from build123d import *

# Parameters (mm, degrees)
SKETCH1_R           = 1.6
BOSS_EXTRUDE1_DEPTH = 6
SKETCH2_W           = 138.2
SKETCH2_H           = 67.6
SKETCH2_R           = 2.5
BOSS_EXTRUDE2_DEPTH = 3.2
FILLET1_R           = 6
FILLET2_R           = 5
FILLET3_R           = 5


with BuildPart() as part:
    # Sketch1 → Boss-Extrude1 (new body)
    with BuildSketch(Plane.XY):
        with BuildLine():
            Line((0, 21.6), (-6, 21.6))
            ThreePointArc((-6, 21.6), (-9.6, 18), (-6, 14.4))
            Line((-6, 14.4), (0, 14.4))
            Line((0, 14.4), (0, 0))
            Line((0, 0), (102.2, 0))
            Line((102.2, 0), (102.2, 46))
            Line((102.2, 46), (108.2, 46))
            ThreePointArc((108.2, 46), (111.8, 49.6), (108.2, 53.2))
            Line((108.2, 53.2), (102.2, 53.2))
            Line((102.2, 53.2), (102.2, 67.6))
            Line((102.2, 67.6), (0, 67.6))
            Line((0, 67.6), (0, 21.6))
        make_face()
        with Locations((-6, 18)):
            Circle(SKETCH1_R, mode=Mode.SUBTRACT)
        with BuildLine():
            Line((94.706674091, 2.5), (7.493325909, 2.5))
            ThreePointArc((7.493325909, 2.5), (7.045584412, 7.045584412), (2.5, 7.493325909))
            Line((2.5, 7.493325909), (2.5, 65.1))
            Line((2.5, 65.1), (99.7, 65.1))
            Line((99.7, 65.1), (99.7, 57.093325909))
            ThreePointArc((99.7, 57.093325909), (94.1, 54.1), (99.7, 51.106674091))
            Line((99.7, 51.106674091), (99.7, 7.493325909))
            ThreePointArc((99.7, 7.493325909), (95.154415588, 7.045584412), (94.706674091, 2.5))
        make_face(mode=Mode.SUBTRACT)
        with Locations((108.2, 49.6)):
            Circle(SKETCH1_R, mode=Mode.SUBTRACT)
        with Locations((4.5, 4.5)):
            Circle(SKETCH1_R, mode=Mode.SUBTRACT)
        with Locations((97.7, 4.5)):
            Circle(SKETCH1_R, mode=Mode.SUBTRACT)
        with Locations((97.7, 54.1)):
            Circle(SKETCH1_R, mode=Mode.SUBTRACT)
    extrude(amount=BOSS_EXTRUDE1_DEPTH)

    # Sketch2 → Boss-Extrude2 (add)
    with BuildSketch(Plane(origin=(0, 0, 0), x_dir=(-1, 0, 0), z_dir=(0, 0, -1))):
        with Locations((-51.1, 33.8)):
            Rectangle(SKETCH2_W, SKETCH2_H)
        with Locations((-112.2, 59.6)):
            Circle(SKETCH2_R, mode=Mode.SUBTRACT)
        with Locations((-112.2, 8)):
            Circle(SKETCH2_R, mode=Mode.SUBTRACT)
        with Locations(Location((10, 8, 0), (0, 0, 180))):
            Circle(SKETCH2_R, mode=Mode.SUBTRACT)
        with Locations(Location((10, 59.6, 0), (0, 0, 180))):
            Circle(SKETCH2_R, mode=Mode.SUBTRACT)
    extrude(amount=BOSS_EXTRUDE2_DEPTH)

    # Fillet1
    fillet1_edges = [part.edges().sort_by_distance(p)[0] for p in [
        (120.2, 67.6, -1.6),
        (120.2, 0, -1.6),
        (-18, 0, -1.6),
        (-18, 67.6, -1.6),
    ]]
    fillet(fillet1_edges, radius=FILLET1_R)

    # Fillet2
    fillet2_edges = [part.edges().sort_by_distance(p)[0] for p in [
        (99.7, 51.106674091, 3),
        (99.7, 57.093325909, 3),
    ]]
    fillet(fillet2_edges, radius=FILLET2_R)

    # Fillet3
    fillet3_edges = [part.edges().sort_by_distance(p)[0] for p in [
        (7.493325909, 2.5, 3),
        (94.706674091, 2.5, 3),
        (99.7, 7.493325909, 3),
        (2.5, 7.493325909, 3),
    ]]
    fillet(fillet3_edges, radius=FILLET3_R)


solid = part.part
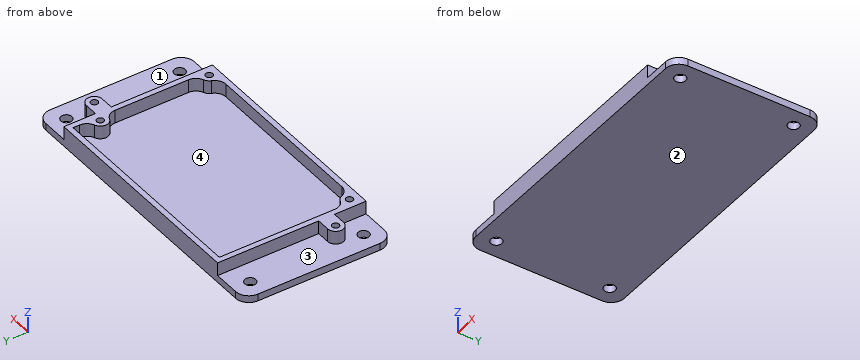
Source: CAD feature listing. Evaluate the final solid. Frame: model axes, mm. Face numbers are marked on the shaded views. A direction names the side the tool comes from. Round coordinates to 2 decimals unless told otherwise and drop trailing zeros. Loops run counter-clockwise (first coordinate to the right, second up) from the corner with the lowest first, then second, coordinate; pieces in that order, holes last.
Q1. Section B-B, the plane z = 3. State how many separate pieces and enclosed holes the cut face has, plus the area to 3 significant figures.
Q2. Section D-D, the plane y = 59.6. Return loops of the section in (x, z), plus the area to 3 significant figures.
Q3. Section C-C, the plane y = 18. Return loops of the section in (x, z).
Q4. Ray query, line 1 (Y direction, x = 112.2, z = -0.95); line 2 (Y direction, x = -6, z = 1.75); line 3 (X direction, y = 63, z = 4). Return the intervals inside material, ascending.
Q5. Section A-A, the plane x = -3. Return loops of the section in (y, z), plus the area to 3 significant figures.
Q6. Mould query, pull axis X, two halves, no side actions, for the marked faces 3 and 4. Classes: pulls with the +X half, pulls with the -X half, needs draft (parallel to the pull), parting line crosses it, or undercut.
Q7. Access query for the marked faces 1 and 2. Directions: +Z, -Z, +X, -X, +Y, -Y. A direction counts if a zero-diameter tool reaches every point of the face in a straight line with its end or side. Return the directions, or none.
Q8. First-contact query: P1, Ø1, axis at x = 97.5, y = 53.5, coming from the +Z side; P2, Ø3, axis at x = 112.2, y = 8, coming from the -Z side; P3, Ø2.5, axis at x = 108, y = 49, coming from the +Z side; P4, Ø3, axis at y = 44, z = 3, coming from the -X side. Flat tips, straight axial feed; report the tip coordinate or a pass-through.
Solutions:
1. separate pieces: 1
1. enclosed holes: 6
1. area: 1,020 mm2
2. outline: (-18, -3.2) - (-12.5, -3.2) - (-12.5, 0) - (-18, 0) - close; (-7.5, -3.2) - (109.7, -3.2) - (109.7, 0) - (102.2, 0) - (102.2, 6) - (99, 6) - (99, 0) - (2.5, 0) - (2.5, 6) - (0, 6) - (0, 0) - (-7.5, 0) - close; (114.7, -3.2) - (120.2, -3.2) - (120.2, 0) - (114.7, 0) - close
2. area: 444 mm2
3. outline: (-18, -3.2) - (120.2, -3.2) - (120.2, 0) - (102.2, 0) - (102.2, 6) - (99.7, 6) - (99.7, 0) - (2.5, 0) - (2.5, 6) - (-4.4, 6) - (-4.4, 0) - (-7.6, 0) - (-7.6, 6) - (-9.6, 6) - (-9.6, 0) - (-18, 0) - close
4. line 1: y = 0 to 5.5, 10.5 to 57.1, 62.1 to 67.6
4. line 2: y = 14.4 to 16.4, 19.6 to 21.6
4. line 3: x = 0 to 2.5, 99.7 to 102.2
5. outline: (0, -3.2) - (67.6, -3.2) - (67.6, 0) - (21.6, 0) - (21.6, 6) - (14.4, 6) - (14.4, 0) - (0, 0) - close
5. area: 260 mm2
6. face 3: needs draft
6. face 4: undercut
7. face 1: +Z, +X
7. face 2: -Z, +X, -X, +Y, -Y
8. P1: stops at z = 0
8. P2: passes through
8. P3: stops at z = 6
8. P4: stops at x = 0
